Check sheet for the modelled part. Datum: model origin and axes. Units: mm. A direction names the side the tool comes from. Give positions to 0.01 mm unless a question says otherwise; leave off trailing zeros. Loops run counter-clockwise (first coordinate to the right, second up) from the corner with the lowest first, then second, coordinate; pieces in that order, holes last.
```python
from build123d import *

# Parameters (mm, degrees)
F1_DEPTH = 35
F2_T     = -1.5
F4_D     = 6
F4_DEPTH = 31.4714761276
F5_D     = 6


with BuildPart() as f1:
    # F0 (on Front) → F1 (new body)
    with BuildSketch(Plane.XZ):
        Polygon((-31.4704761276, 48.409471255), (-25, 24.2613255978), (25, 24.2613255978), (31.4704761276, 48.409471255), align=None)
    extrude(amount=F1_DEPTH)

    # F2
    f2_openings = [f1.faces().sort_by_distance(p)[0] for p in [
        (0, -17.5, 48.409471),
    ]]
    offset(amount=F2_T, openings=f2_openings)

    # F4 (through all, one way)
    with BuildSketch(Plane.YZ):
        with Locations((-17.5, 36.3353984264)):
            Circle(F4_D / 2)
    extrude(amount=-F4_DEPTH, mode=Mode.SUBTRACT)

    # F5 (through all)
    with Locations(Plane(origin=(0, 0, 0), x_dir=(0, 1, 0), z_dir=(-1, 0, 0))):
        with Locations((-17.5, -36.3353984264)):
            Hole(F5_D / 2)


solid = f1.part
```
(1) Section check B-B on y = -17.5. Record the boundary of the cut face in (x, z), plus the area to 3 significant figures.
(2) Section check D-D on y = -3.5. Record the boundary of the cut face in (x, z), plus the area to 3 significant figures.
(3) Section check A-A on z = 38.25. Record the boundary of the cut face in (x, y), plus the area to 3 significant figures.
(4) Material ranges on line 1 (Y direction, x = -16, z = 31); line 2 (Z direction, x = 9, y = -19.5); line 3 (X direction, y = -16.5, z = 27.25), recorded low to high.
(5) Gauge pin test, flat ends, axial feed: pin 1 Ø4 at (x, y) = (16, -20) entering from +Z; pin 2 Ø1.5 at (y, z) = (-7, 34) entering from +X; pin 3 Ø9.5 at (y, z) = (-17.5, 36.34) entering from +X. Record the tip position at first contact, or that the pin passes through.
(6) Access from +Z, -Z, +X, -X, +Y, -Y to the whole of each face (thin tool, end or side, straight path). Record for faces 5 (the face through (0, -33.5, 37)), 6 (the face through (27.82, -18.88, 39)).
(7) Release check for a two-part mould opening along Z. For faces 1 (the face through (2, -34, 48.409)), 2 (the face through (-27.43, -19.88, 34.51)), 3 (the face through (0, 0, 37)), 4 (the face through (0, -17, 24.261)) record: pulls with the +Z half, pulls with the -Z half, needs draft (parallel to the pull), parting line crosses it, or undercut.
(8) Section check C-C on x = 19. Record the boundary of the cut face in (y, z).
Computed values:
1. outline: (-31.47, 48.41) - (-29.04, 39.34) - (-27.49, 39.34) - (-29.92, 48.41) - close; (-27.43, 33.34) - (-25, 24.26) - (25, 24.26) - (27.43, 33.34) - (25.88, 33.34) - (23.85, 25.76) - (-23.85, 25.76) - (-25.88, 33.34) - close; (27.49, 39.34) - (29.04, 39.34) - (31.47, 48.41) - (29.92, 48.41) - close
1. area: 127 mm2
2. outline: (-31.47, 48.41) - (-25, 24.26) - (25, 24.26) - (31.47, 48.41) - (29.92, 48.41) - (23.85, 25.76) - (-23.85, 25.76) - (-29.92, 48.41) - close
2. area: 146 mm2
3. outline: (-28.75, -35) - (28.75, -35) - (28.75, -19.81) - (27.2, -19.81) - (27.2, -33.5) - (-27.2, -33.5) - (-27.2, -19.81) - (-28.75, -19.81) - close; (-28.75, -15.19) - (-27.2, -15.19) - (-27.2, -1.5) - (27.2, -1.5) - (27.2, -15.19) - (28.75, -15.19) - (28.75, 0) - (-28.75, 0) - close
3. area: 258 mm2
4. line 1: y = -35 to -33.5, -1.5 to 0
4. line 2: z = 24.26 to 25.76
4. line 3: x = -25.8 to -24.25, 24.25 to 25.8
5. pin 1: stops at z = 25.76
5. pin 2: stops at x = 27.81
5. pin 3: stops at x = 29.51
6. face 5: +Z
6. face 6: +X, -X
7. face 1: pulls with the +Z half
7. face 2: undercut
7. face 3: needs draft
7. face 4: pulls with the -Z half
8. outline: (-35, 24.26) - (0, 24.26) - (0, 48.41) - (-1.5, 48.41) - (-1.5, 25.76) - (-33.5, 25.76) - (-33.5, 48.41) - (-35, 48.41) - close
